Autodesk Inventor part; units mm, degrees
ref_plane "YZ Plane" through (0, 0, 0) normal (1, 0, 0) x (0, 1, 0)
ref_plane "XZ Plane" through (0, 0, 0) normal (0, 1, 0) x (-1, 0, 0)
ref_plane "XY Plane" through (0, 0, 0) normal (0, 0, 1) x (1, 0, 0)
sketch "Sketch1" plane through (0, 0, 0) normal (0, 0, 1) x (1, 0, 0)
  line L0 (0, 0) -> (20, 0)
  line L1 (20, 0) -> (20, 40.5)
  line L2 (20, 40.5) -> (0, 40.5)
  line L3 (0, 40.5) -> (0, 0)
  circle A0 centre (10, 0) radius 30
  circle A1 centre (10, 0) radius 10
  line L4 (-8, 0) -> (28, 0)
  line L5 (28, 0) -> (28, 100)
  line L6 (28, 100) -> (-8, 100)
  line L7 (-8, 100) -> (-8, 0)
  circle A2 centre (10, 100) radius 30
  circle A3 centre (10, 100) radius 10
  point P0 (28, 24)
  point P1 (28, 76)
  point P2 (-8, 76)
  point P3 (-8, 24)
  dimension "d2" = 20
  dimension "d3" = 40.5
  dimension "d4" = 60
  dimension "d5" = 20
  dimension "d6" = 36
  dimension "d7" = 100
  dimension "d8" = 60
  dimension "d9" = 20
extrude "Extrusion1" add sketch "Sketch1" along normal blind 10 contours L4 L7 A0 L3 | L3 A0 L1 A1 | A1 L4 L5 A0 L7 | L1 A0 L5 L4 | A0 L7 A2 L5 L1 L2 L3 | L3 L2 L1 A0 | A2 L5 L6 A3 L7 | L7 L6 A3 L5 A2
fillet "Fillet1" radius 2 8 edges at (10, 130, 10) (28, 50, 10) (-8, 50, 10) (10, -30, 10) (10, 130, 0) (28, 50, 0) (10, -30, 0) (-8, 50, 0)
sketch "Sketch2" plane through (0, 0, 10) normal (0, 0, 1) x (1, 0, 0)
  line L0 (0, 0) -> (20, 0)
  line L1 (20, 0) -> (20, 40.5)
  line L2 (20, 40.5) -> (0, 40.5)
  line L3 (0, 40.5) -> (0, 0)
  dimension "d13" = 20
  dimension "d14" = 40.5
extrude "Extrusion2" cut sketch "Sketch2" against normal blind 10.6375
properties part number "2nd arm"
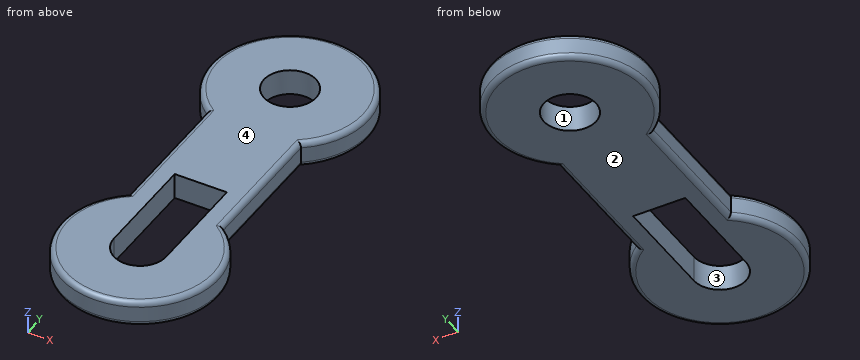
Part model, mm, in its own coordinate system. Face numbers are marked on the shaded views. A direction names the side the tool comes from. Coordinates: 2 decimals unless noted, no trailing zeros. Loops run counter-clockwise (first coordinate to the right, second up) from the corner with the lowest first, then second, coordinate; pieces in that order, holes last. Notation, with made-up numbers: M 86.5,45.5 L 135.5,45.5 A13 cw 135.5,69.5 Z; hole C 6.25,56.5 d4. An arc over 180 degrees is marked long. Use a Markdown table: item, result. Add a question column.
Q1. Probe L1, parallel to Y at x = 10, z = 4; L2, parallel to X at y = 100, z = 3.25; L3, parallel to Y at x = 11, z = 1. List the from-to ranges inside material, lowest first.
Q2. Cut at C-C (z = 4.25). Write the cut outline in (x, y), and give its area (3 significant figures).
Q3. Mould opens along X. For the marked faces 1 and 2 say: +X half, -X half, draft (parallel to the pull), parting line (faces both ways), or undercut.
Q4. Cut at A-A (y = 34). Write the cut outline in (x, z).
Q5. Which spindle directions (+Z, -Z, +X, -X, +Y, -Y) get a long thin tool onto all of the face, cutting with end or side? Do the marked faces 3 and 4. Say none if no direction does.
Q6. Cut at D-D (y = 100). Write the cut outline in (x, z).
Q7. Pin check, flat tips, straight feed: P1, Ø1.5, axis at x = 31, z = 2, coming from the +Y side; P2, Ø5, axis at y = 56, z = 5, coming from the -X side; P3, Ø3, axis at x = 6.5, z = 6.5, coming from the -Y side. Stop position of each tip, or through.
Q8. Cut at B-B (x = 10). Write the cut outline in (y, z), and give its area (3 significant figures).
Worked out:
| question | item | result |
|---|---|---|
| 1 | L1 | y = -30 to -10, 40.5 to 90, 110 to 130 |
| 1 | L2 | x = -20 to 0, 20 to 40 |
| 1 | L3 | y = -29.72 to -9.95, 40.5 to 90.05, 109.95 to 129.72 |
| 2 | outline | M -8,24 A30 ccw long 28,24 L 28,76 A30 ccw long -8,76 Z; hole M 0,0 A10 ccw 20,0 L 20,40.5 L 0,40.5 Z; hole C 10,100 d20 |
| 2 | area | 5,950 mm2 |
| 3 | face 1 | undercut |
| 3 | face 2 | draft |
| 4 | outline | M -8,2 A2 ccw -6,0 L 0,0 L 0,10 L -6,10 A2 ccw -8,8 Z; M 20,0 L 26,0 A2 ccw 28,2 L 28,8 A2 ccw 26,10 L 20,10 Z |
| 5 | face 3 | +Z, -Z |
| 5 | face 4 | +Z, +X, -X, +Y, -Y |
| 6 | outline | M -20,2 A2 ccw -18,0 L 0,0 L 0,10 L -18,10 A2 ccw -20,8 Z; M 20,0 L 38,0 A2 ccw 40,2 L 40,8 A2 ccw 38,10 L 20,10 Z |
| 7 | P1 | stops at y = 122.13 |
| 7 | P2 | stops at x = -8 |
| 7 | P3 | stops at y = -29.93 |
| 8 | outline | M -30,2 A2 ccw -28,0 L -10,0 L -10,10 L -28,10 A2 ccw -30,8 Z; M 40.5,0 L 90,0 L 90,10 L 40.5,10 Z; M 110,0 L 128,0 A2 ccw 130,2 L 130,8 A2 ccw 128,10 L 110,10 Z |
| 8 | area | 892 mm2 |
